Part print with two shaded views. Sizes in mm from the minimum x, y, z corner. Coordinates: 2 decimals unless noted, no trailing zeros. Loops run counter-clockwise (first coordinate to the right, second up) from the corner with the lowest first, then second, coordinate; pieces in that order, holes last. Notation, with made-up numbers: (41.25, 5) -> (63.25, 5) arc R21 ccw to (63.25, 23) -> close; hole circle Ø5 at (52, 73.25). An arc over 180 degrees is marked (long way). Use one line per item in the form item = value.
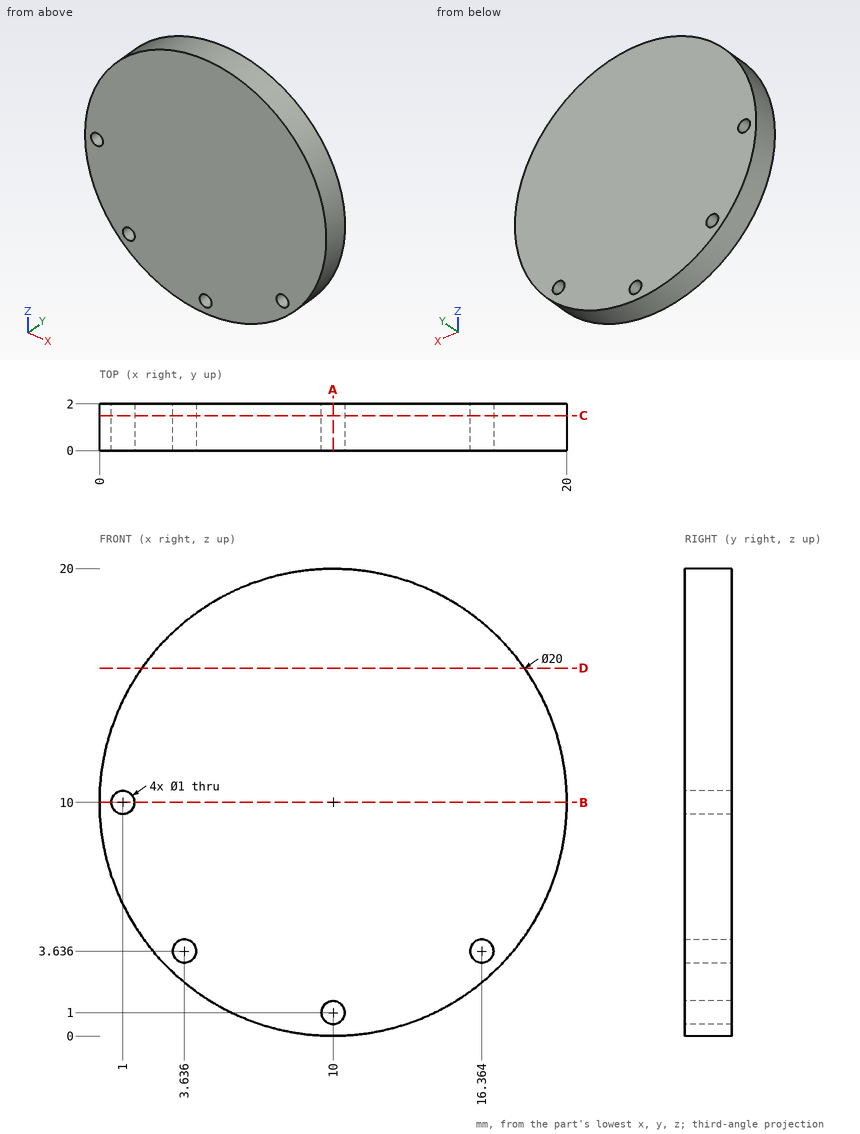
Q1. Band-saw the part on A-A, the plane x = 10. Write the cut outline in (y, z), and give its area (3 significant figures).
Result:
outline = (0, 0) -> (2, 0) -> (2, 0.5) -> (0, 0.5) -> close; (0, 1.5) -> (2, 1.5) -> (2, 20) -> (0, 20) -> close
area = 38.0 mm2
Q2. Band-saw the part on B-B, the plane z = 10. Write the cut outline in (x, y), and give its area (3 significant figures).
Result:
outline = (0, 0) -> (0.5, 0) -> (0.5, 2) -> (0, 2) -> close; (1.5, 0) -> (20, 0) -> (20, 2) -> (1.5, 2) -> close
area = 38.0 mm2
Q3. Band-saw the part on C-C, the plane y = 1.5. Write the cut outline in (x, z), and give its area (3 significant figures).
Result:
outline = circle Ø20 at (10, 10); hole circle Ø1 at (1, 10); hole circle Ø1 at (3.64, 3.64); hole circle Ø1 at (10, 1); hole circle Ø1 at (16.36, 3.64)
area = 311 mm2
Q4. Pin check, flat tips, straight feed: pin 1 Ø1 at (x, y) = (16.5, 1) entering from +Z; pin 2 Ø1 at (y, z) = (1.5, 14.5) entering from -X. Stop position of each tip, or through.
Result:
pin_1 = 18
pin_2 = 0.83
Q5. Wall check: line 1 along Z through (x, y) = (10, 1.1); line 2 along X through (y, z) = (0.35, 1.25); line 3 along Z through (x, y) = (1, 0.85). Give the ranges that are in metal, low to high.
Result:
line_1 = 0 to 0.5, 1.5 to 20
line_2 = 5.16 to 9.57, 10.43 to 14.84
line_3 = 5.64 to 9.5, 10.5 to 14.36
Q6. Band-saw the part on D-D, the plane z = 15.75. Write the cut outline in (x, y).
Result:
outline = (1.82, 0) -> (18.18, 0) -> (18.18, 2) -> (1.82, 2) -> close
